Geometry check sheet. Reference: the model listing, model coordinates, mm. Give positions to 0.01 mm unless a question says otherwise; leave off trailing zeros. Write each loop counter-clockwise with the first axis right and the second up, starting at its lowest first coordinate (ties: lowest second). Pieces come first, ordered by that corner, then holes. Notation, with made-up numbers: M 69,-35 L 96,-35 A19 cw 96,-29 Z; hole C 4.25,1.25 d8. An arc over 180 degrees is marked long. One line per item, written item: value. Start each with the question number.
1. Cross-section at D-D on x = 18.5. Record the cut outline in (y, z), then the cut area to 3 significant figures.
2. Gauge pin test, flat ends, axial feed: pin 1 (1.8 mm diameter, centred on x = 270.75, z = 51, fed in from +Y); pin 2 (5 mm diameter, centred on x = 80, z = -72.5, fed in from +Y); pin 3 (1 mm diameter, centred on x = 237, y = 1.5, fed in from -Z); pin 4 (4 mm diameter, centred on x = 131.27, z = 51.27, fed in from +Y). Record the tip position at first contact, or that the pin passes through.
3. Cross-section at A-A on x = 208.5. Record the cut outline in (y, z), then the cut area to 3 significant figures.
4. Cross-section at B-B on x = 89.5. Record the cut outline in (y, z), then the cut area to 3 significant figures.
5. Scan lines: line 1 (Z direction, x = 270.75, y = 1.05); line 2 (Z direction, x = 163.5, y = 0.7); line 3 (Z direction, x = 165.5, y = 0.65). Record each from-to range of solid material in increasing order.
6. Cross-section at C-C on z = 44. Record the cut outline in (x, y), then the cut area to 3 significant figures.
from build123d import *
from OCP.BRepFilletAPI import BRepFilletAPI_MakeChamfer

# Parameters (mm, degrees)
SKETCH1_R           = 20
SKETCH1_R_2         = 1.5
SKETCH1_R_3         = 2
SKETCH1_R_4         = 1.4
BOSS_EXTRUDE1_DEPTH = 3.2
CHAMFER1_SIZE       = 1.2
CHAMFER1_SIZE2      = 1.997135379


with BuildPart() as part:
    # Sketch1 → Boss-Extrude1 (new body)
    with BuildSketch(Plane(origin=(0, 0, 0), x_dir=(1, 0, 0), z_dir=(0, 1, 0))):
        with BuildLine():
            Line((283, 55), (283, -55))
            ThreePointArc((283, -55), (281.535533906, -58.535533906), (278, -60))
            Line((278, -60), (133.66563146, -60))
            ThreePointArc((133.66563146, -60), (132.967201164, -60.125914857), (132.35671362, -60.487804878))
            ThreePointArc((132.35671362, -60.487804878), (0, 0), (132.35671362, 60.487804878))
            ThreePointArc((132.35671362, 60.487804878), (132.967201164, 60.125914857), (133.66563146, 60))
            Line((133.66563146, 60), (278, 60))
            ThreePointArc((278, 60), (281.535533906, 58.535533906), (283, 55))
        make_face()
        with Locations(Location((80, 0, 0), (0, 0, 270))):
            Circle(SKETCH1_R, mode=Mode.SUBTRACT)
        with Locations(Location((7.5, 0, 0), (0, 0, 270))):
            Circle(SKETCH1_R_2, mode=Mode.SUBTRACT)
        with Locations(Location((28.734758364, 51.265241636, 0), (0, 0, 270))):
            Circle(SKETCH1_R_2, mode=Mode.SUBTRACT)
        with Locations(Location((80, 72.5, 0), (0, 0, 270))):
            Circle(SKETCH1_R_2, mode=Mode.SUBTRACT)
        with Locations(Location((131.265241636, 51.265241636, 0), (0, 0, 270))):
            Circle(SKETCH1_R_2, mode=Mode.SUBTRACT)
        with Locations(Location((131.265241636, -51.265241636, 0), (0, 0, 270))):
            Circle(SKETCH1_R_2, mode=Mode.SUBTRACT)
        with Locations(Location((80, -72.5, 0), (0, 0, 270))):
            Circle(SKETCH1_R_2, mode=Mode.SUBTRACT)
        with Locations(Location((28.734758364, -51.265241636, 0), (0, 0, 270))):
            Circle(SKETCH1_R_2, mode=Mode.SUBTRACT)
        with Locations(Location((30.5, 0, 0), (0, 0, 270))):
            Circle(SKETCH1_R_3, mode=Mode.SUBTRACT)
        with Locations(Location((270.75, 51, 0), (0, 0, 270))):
            Circle(SKETCH1_R_2, mode=Mode.SUBTRACT)
        with Locations(Location((270.75, -51, 0), (0, 0, 270))):
            Circle(SKETCH1_R_2, mode=Mode.SUBTRACT)
        with Locations(Location((163.5, 20, 0), (0, 0, 270))):
            Circle(SKETCH1_R_4, mode=Mode.SUBTRACT)
        with Locations(Location((163.5, -20, 0), (0, 0, 270))):
            Circle(SKETCH1_R_4, mode=Mode.SUBTRACT)
        with Locations(Location((157.75, 6.8, 0), (0, 0, 270))):
            Circle(SKETCH1_R_2, mode=Mode.SUBTRACT)
        with Locations(Location((200.75, 6.8, 0), (0, 0, 270))):
            Circle(SKETCH1_R_2, mode=Mode.SUBTRACT)
        with Locations(Location((80, 49.5, 0), (0, 0, 270))):
            Circle(SKETCH1_R_3, mode=Mode.SUBTRACT)
        with Locations(Location((129.5, 0, 0), (0, 0, 270))):
            Circle(SKETCH1_R_3, mode=Mode.SUBTRACT)
        with Locations(Location((80, -49.5, 0), (0, 0, 270))):
            Circle(SKETCH1_R_3, mode=Mode.SUBTRACT)
        with BuildLine():
            Line((157.5, -29), (257.5, -29))
            ThreePointArc((257.5, -29), (259, -27.5), (257.5, -26))
            Line((257.5, -26), (157.5, -26))
            ThreePointArc((157.5, -26), (156, -27.5), (157.5, -29))
        make_face(mode=Mode.SUBTRACT)
        with BuildLine():
            Line((257.5, 26), (157.5, 26))
            ThreePointArc((157.5, 26), (156, 27.5), (157.5, 29))
            Line((157.5, 29), (257.5, 29))
            ThreePointArc((257.5, 29), (259, 27.5), (257.5, 26))
        make_face(mode=Mode.SUBTRACT)
    extrude(amount=BOSS_EXTRUDE1_DEPTH)

    # Chamfer1: one chamfer whose edges measure the first distance from different faces: ONE call of the kernel's chamfer builder (chamfer() names one face for all edges)
    chamfer1_edges_1 = [part.edges().sort_by_distance(p)[0] for p in [
        (28.734758364, 3.2, -52.765241636),
        (80, 3.2, -74),
        (131.265241636, 3.2, -52.765241636),
        (131.265241636, 3.2, 49.765241636),
        (80, 3.2, 71),
        (28.734758364, 3.2, 49.765241636),
        (270.75, 3.2, -52.5),
        (7.5, 3.2, -1.5),
    ]]
    chamfer1_side_1 = [part.faces().sort_by_distance(p)[0] for p in [
        (141.32803895, 3.2, 0.002840635),
    ]]
    chamfer1_edges_2 = [part.edges().sort_by_distance(p)[0] for p in [
        (270.75, 3.2, 49.5),
    ]]
    chamfer1_side_2 = [part.faces().sort_by_distance(p)[0] for p in [
        (270.75, 1.6, 49.5),
    ]]
    chamfer1 = BRepFilletAPI_MakeChamfer(part.part.solid().wrapped)
    for e in chamfer1_edges_1:
        chamfer1.Add(CHAMFER1_SIZE, CHAMFER1_SIZE2, e.wrapped, chamfer1_side_1[0].wrapped)  # the first distance lies on this face
    for e in chamfer1_edges_2:
        chamfer1.Add(CHAMFER1_SIZE, CHAMFER1_SIZE2, e.wrapped, chamfer1_side_2[0].wrapped)  # the first distance lies on this face
    add(Compound.cast(chamfer1.Shape()), mode=Mode.REPLACE)


solid = part.part
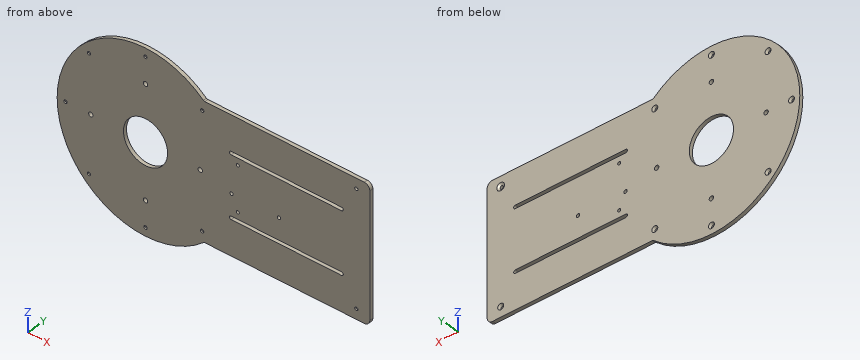
Report:
1. outline: M 0,-51.16 L 3.2,-51.16 L 3.2,51.16 L 0,51.16 Z
1. area: 327 mm^2
2. pin 1: passes through
2. pin 2: stops at y = 2.87
2. pin 3: stops at z = -60
2. pin 4: stops at y = 2.05
3. outline: M 0,-60 L 3.2,-60 L 3.2,-29 L 0,-29 Z; M 0,-26 L 3.2,-26 L 3.2,26 L 0,26 Z; M 0,29 L 3.2,29 L 3.2,60 L 0,60 Z
3. area: 365 mm^2
4. outline: M 0,-79.43 L 3.2,-79.43 L 3.2,-17.6 L 0,-17.6 Z; M 0,17.6 L 3.2,17.6 L 3.2,79.43 L 0,79.43 Z
4. area: 396 mm^2
5. line 1: z = -60 to -52.5, -49.5 to 49.5, 52.5 to 60
5. line 2: z = -60 to -29, -26 to -21.4, -18.6 to 18.6, 21.4 to 26, 29 to 60
5. line 3: z = -60 to -29, -26 to 26, 29 to 60
6. outline: M 13.19,0 L 283,0 L 283,3.2 L 13.19,3.2 Z
6. area: 863 mm^2
